```python
from build123d import *

# Parameters (mm, degrees)
SKETCH_1_R             = 35
EXTRUDE_1_DEPTH        = 102
SKETCH_2_R             = 20
EXTRUDE_2_DEPTH        = 3
SKETCH_3_R             = 7
EXTRUDE_3_DEPTH        = 32
SKETCH_4_W             = 72
SKETCH_4_H             = 72
EXTRUDE_4_DEPTH        = 21
CHAMFER_1_SIZE         = 5
SKETCH_5_R             = 2
CUT_EXTRUDE_1_DEPTH    = 10
CHAMFER_2_SIZE         = 0.5
SKETCH_6_R             = 25
CUT_EXTRUDE_2_DEPTH    = 9
SKETCH_7_R             = 8
CUT_EXTRUDE_3_DEPTH    = 9
SKETCH_9_R             = 2.5
CUT_EXTRUDE_4_DEPTH    = 9
SKETCH_10_R            = 2.5
CUT_EXTRUDE_5_DEPTH    = 19
EXTRUDE_1_2_DEPTH      = 1
EXTRUDE_1_2_DEPTH_BACK = 2
SKETCH_13_R            = 7.497429265
SKETCH_13_R_2          = 6
EXTRUDE_2_2_DEPTH      = 9
CUT_EXTRUDE_START      = -19
SKETCH_14_R            = 6
CUT_EXTRUDE_6_DEPTH    = 19


with BuildPart() as part:
    # Эскиз1 → Extrude 1 (new body)
    with BuildSketch(Plane(origin=(0, 0, 0), x_dir=(1, 0, 0), z_dir=(0, 1, 0))):
        with Locations(Location((0, 0, 0), (0, 0, 270))):
            Circle(SKETCH_1_R)
    extrude(amount=EXTRUDE_1_DEPTH)

    # Эскиз2 → Extrude 2 (add)
    with BuildSketch(Plane(origin=(0, 102, 0), x_dir=(1, 0, 0), z_dir=(0, 1, 0))):
        with Locations(Location((0, 0, 0), (0, 0, 270))):
            Circle(SKETCH_2_R)
    extrude(amount=EXTRUDE_2_DEPTH)

    # Эскиз3 → Вытянуть3 (add)
    with BuildSketch(Plane(origin=(0, 105, 0), x_dir=(1, 0, 0), z_dir=(0, 1, 0))):
        with Locations(Location((0, 0, 0), (0, 0, 270))):
            Circle(SKETCH_3_R)
    extrude(amount=EXTRUDE_3_DEPTH)

    # Эскиз4 → Вытянуть4 (add)
    with BuildSketch(Plane.XZ):
        Rectangle(SKETCH_4_W, SKETCH_4_H)
    extrude(amount=EXTRUDE_4_DEPTH)

    # Фаска1
    chamfer_1_edges = [part.edges().sort_by_distance(p)[0] for p in [
        (-36, -10.5, 36),
        (-36, -10.5, -36),
        (36, -10.5, -36),
        (36, -10.5, 36),
    ]]
    chamfer(chamfer_1_edges, length=CHAMFER_1_SIZE)

    # Эскиз5 → Вырез-Вытянуть1 (cut)
    with BuildSketch(Plane(origin=(0, 102, 0), x_dir=(1, 0, 0), z_dir=(0, 1, 0))):
        with Locations(Location((-18.384776311, 18.384776311, 0), (0, 0, 270))):
            Circle(SKETCH_5_R)
        with Locations(Location((18.384776311, 18.384776311, 0), (0, 0, 270))):
            Circle(SKETCH_5_R)
        with Locations(Location((-18.384776311, -18.384776311, 0), (0, 0, 270))):
            Circle(SKETCH_5_R)
        with Locations(Location((18.384776311, -18.384776311, 0), (0, 0, 270))):
            Circle(SKETCH_5_R)
    extrude(amount=-CUT_EXTRUDE_1_DEPTH, mode=Mode.SUBTRACT)

    # Фаска2
    chamfer_2_edges = [part.edges().sort_by_distance(p)[0] for p in [
        (0, 102, -35),
        (-18.384776311, 102, -20.384776311),
        (18.384776311, 102, -20.384776311),
        (-18.384776311, 102, 16.384776311),
        (0, 102, -20),
        (18.384776311, 102, 16.384776311),
    ]]
    chamfer(chamfer_2_edges, length=CHAMFER_2_SIZE)

    # Эскиз6 → Вырез-Вытянуть2 (cut)
    with BuildSketch(Plane.XZ.offset(21)):
        with Locations(Location((0, 0, 0), (0, 0, 270))):
            Circle(SKETCH_6_R)
    extrude(amount=-CUT_EXTRUDE_2_DEPTH, mode=Mode.SUBTRACT)

    # Эскиз7 → Вырез-Вытянуть3 (cut)
    with BuildSketch(Plane.XZ.offset(12)):
        with Locations(Location((0, 0, 0), (0, 0, 270))):
            Circle(SKETCH_7_R)
    extrude(amount=-CUT_EXTRUDE_3_DEPTH, mode=Mode.SUBTRACT)

    # Эскиз9 → Вырез-Вытянуть4 (cut)
    with BuildSketch(Plane.XZ.offset(21)):
        with Locations(Location((-24.748737342, 24.748737342, 0), (0, 0, 270))):
            Circle(SKETCH_9_R)
        with Locations(Location((24.748737342, 24.748737342, 0), (0, 0, 270))):
            Circle(SKETCH_9_R)
        with Locations(Location((-24.748737342, -24.748737342, 0), (0, 0, 270))):
            Circle(SKETCH_9_R)
        with Locations(Location((24.748737342, -24.748737342, 0), (0, 0, 270))):
            Circle(SKETCH_9_R)
    extrude(amount=-CUT_EXTRUDE_4_DEPTH, mode=Mode.SUBTRACT)

    # Эскиз10 → Вырез-Вытянуть5 (cut)
    with BuildSketch(Plane(origin=(0, 137, 0), x_dir=(1, 0, 0), z_dir=(0, 1, 0))):
        with Locations(Location((0, 0, 0), (0, 0, 270))):
            Circle(SKETCH_10_R)
    extrude(amount=-CUT_EXTRUDE_5_DEPTH, mode=Mode.SUBTRACT)

    # Эскиз12 → Extrude 1 2 (add, two sides: drawn at the far end of the back side and taken through both)
    with BuildSketch(Plane.XY.offset(-7.151021082).offset(-EXTRUDE_1_2_DEPTH_BACK)):
        with BuildLine():
            Line((2.5, 133.056281521), (2.5, 109.056281521))
            ThreePointArc((2.5, 109.056281521), (0, 106.556281521), (-2.5, 109.056281521))
            Line((-2.5, 109.056281521), (-2.5, 133.056281521))
            ThreePointArc((-2.5, 133.056281521), (0, 135.556281521), (2.5, 133.056281521))
        make_face()
    extrude(amount=EXTRUDE_1_2_DEPTH + EXTRUDE_1_2_DEPTH_BACK)

    # Эскиз13 → Extrude 2 2 (add)
    with BuildSketch(Plane.XZ.offset(3)):
        with Locations(Location((0, 0, 0), (0, 0, 90))):
            Circle(SKETCH_13_R)
        with Locations(Location((0, 0, 0), (0, 0, 90))):
            Circle(SKETCH_13_R_2, mode=Mode.SUBTRACT)
    extrude(amount=EXTRUDE_2_2_DEPTH)

    # Эскиз14 → Вырез-Вытянуть6 (cut)
    with BuildSketch(Plane.XZ.offset(3).offset(CUT_EXTRUDE_START)):
        with Locations(Location((0, 0, 0), (0, 0, 90))):
            Circle(SKETCH_14_R)
    extrude(amount=CUT_EXTRUDE_6_DEPTH, mode=Mode.SUBTRACT)


solid = part.part
```
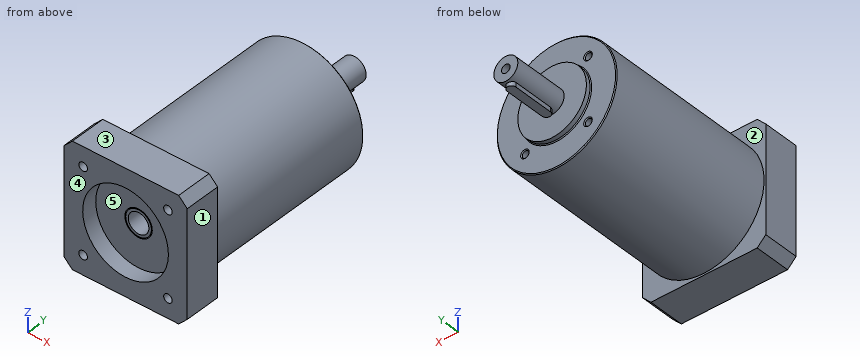
Check sheet for the modelled part. Datum: model origin and axes. Units: mm. Face numbers are marked on the shaded views. A direction names the side the tool comes from. Give positions to 0.01 mm unless a question says otherwise; leave off trailing zeros. Write each loop counter-clockwise with the first axis right and the second up, starting at its lowest first coordinate (ties: lowest second). Pieces come first, ordered by that corner, then holes. Notation, with made-up numbers: (-11.75, -3.75) - (-4.75, -3.75) arc R22 ccw to (-4.75, 10.25) - close; hole circle Ø9 at (53, -34.5). An arc over 180 degrees is marked (long way). Answer as a JSON object with one key per item and string values. Group by question number.
1) Thickness scan on probe 1 along Y at (x, z) = (-15, -21); probe 2 along Y at (x, z) = (13, -11); probe 3 along Z at (x, y) = (1, 48). Record the ranges inside material, lowest first. Write a range as from..to.
2) Access from +Z, -Z, +X, -X, +Y, -Y to the whole of each face (thin tool, end or side, straight path). Record for the marked faces 1 and 2.
3) Depth check by flat-ended pin: P1, Ø8, axis at x = -2, z = -2.5, coming from the -Y side; P2, Ø2.5, axis at x = 0, z = -0.5, coming from the +Y side; P3, Ø1.5, axis at x = 13, y = 52, coming from the -Z side. Enter the tip coordinate at first touch or a pass-through.
4) Release check for a two-part mould opening along Z. For the marked faces 3, 4 and 5 record: pulls with the +Z half, pulls with the -Z half, needs draft (parallel to the pull), parting line crosses it, or undercut.
5) Sectioned sample at B-B (y = 40.5). Record the cut outline in (x, z).
6) Sectioned sample at A-A (y = -9.5). Record the cut outline in (x, z), then the cut area to 3 significant figures.
Geometry results:
{
 "1": {"probe 1": "y = -21..102", "probe 2": "y = -12..105", "probe 3": "z = -34.99..34.99"},
 "2": {"face 1": "+Z, -Z, +X, +Y, -Y", "face 2": "+Y"},
 "3": {"P1": "stops at y = -12", "P2": "stops at y = 118", "P3": "stops at z = -32.79"},
 "4": {"face 3": "pulls with the +Z half", "face 4": "needs draft", "face 5": "undercut"},
 "5": {"outline": "circle Ø70 at (0, 0)"},
 "6": {"outline": "(-36, -31) - (-31, -36) - (31, -36) - (36, -31) - (36, 31) - (31, 36) - (-31, 36) - (-36, 31) - close; circle Ø14.99 at (0, 0); hole circle Ø16 at (0, 0); hole circle Ø12 at (0, 0)", "area": "5,000 mm^2"}
}
